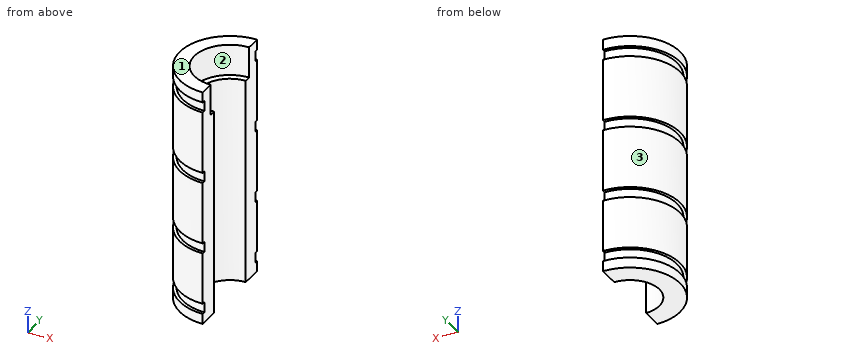
```python
from build123d import *

# Parameters (mm, degrees)
SKETCH1_R           = 24
SKETCH1_R_2         = 14
BOSS_EXTRUDE1_DEPTH = 115
SKETCH2_W           = 30.560484556
SKETCH2_H           = 55.665733052
CUT_EXTRUDE1_DEPTH  = 130
SKETCH3_R           = 17
CUT_EXTRUDE2_DEPTH  = 15
SKETCH4_R           = 29.348690421
SKETCH4_R_2         = 22.5
CUT_EXTRUDE3_DEPTH  = 5
SKETCH5_R           = 32.227537674
SKETCH5_R_2         = 22.5
CUT_EXTRUDE4_DEPTH  = 5
SKETCH6_R           = 32.40953394
SKETCH6_R_2         = 22.5
CUT_EXTRUDE5_DEPTH  = 5
CUT_EXTRUDE6_START  = 5
SKETCH7_R           = 39.356381894
SKETCH7_R_2         = 22.5
CUT_EXTRUDE6_DEPTH  = 5


with BuildPart() as part:
    # Sketch1 → Boss-Extrude1 (new body)
    with BuildSketch(Plane.XY):
        Circle(SKETCH1_R)
        Circle(SKETCH1_R_2, mode=Mode.SUBTRACT)
    extrude(amount=BOSS_EXTRUDE1_DEPTH)

    # Sketch2 → Cut-Extrude1 (cut)
    with BuildSketch(Plane.XY.offset(115)):
        with Locations((15.280242278, -0.503267732)):
            Rectangle(SKETCH2_W, SKETCH2_H)
    extrude(amount=-CUT_EXTRUDE1_DEPTH, mode=Mode.SUBTRACT)

    # Sketch3 → Cut-Extrude2 (cut)
    with BuildSketch(Plane.XY.offset(115)):
        Circle(SKETCH3_R)
    extrude(amount=-CUT_EXTRUDE2_DEPTH, mode=Mode.SUBTRACT)

    # Sketch4 → Cut-Extrude3 (cut)
    with BuildSketch(Plane(origin=(0, 0, 35), x_dir=(-1, 0, 0), z_dir=(0, 0, -1))):
        Circle(SKETCH4_R)
        Circle(SKETCH4_R_2, mode=Mode.SUBTRACT)
    extrude(amount=-CUT_EXTRUDE3_DEPTH, mode=Mode.SUBTRACT)

    # Sketch5 → Cut-Extrude4 (cut)
    with BuildSketch(Plane(origin=(0, 0, 70), x_dir=(-1, 0, 0), z_dir=(0, 0, -1))):
        Circle(SKETCH5_R)
        Circle(SKETCH5_R_2, mode=Mode.SUBTRACT)
    extrude(amount=-CUT_EXTRUDE4_DEPTH, mode=Mode.SUBTRACT)

    # Sketch6 → Cut-Extrude5 (cut)
    with BuildSketch(Plane.XY.offset(105)):
        Circle(SKETCH6_R)
        Circle(SKETCH6_R_2, mode=Mode.SUBTRACT)
    extrude(amount=CUT_EXTRUDE5_DEPTH, mode=Mode.SUBTRACT)

    # Sketch7 → Cut-Extrude6 (cut)
    with BuildSketch(Plane(origin=(0, 0, 10), x_dir=(-1, 0, 0), z_dir=(0, 0, -1)).offset(CUT_EXTRUDE6_START)):
        Circle(SKETCH7_R)
        Circle(SKETCH7_R_2, mode=Mode.SUBTRACT)
    extrude(amount=-CUT_EXTRUDE6_DEPTH, mode=Mode.SUBTRACT)


solid = part.part
```
Geometry: final body of the model. Coordinates: model frame, mm. Face numbers are marked on the shaded views. Give positions to 0.01 mm unless a question says otherwise; leave off trailing zeros. Order: outer loops, then holes, each group sorted by start corner. A loop starts at its lowest first (then second) coordinate and runs counter-clockwise, first axis right, second up. Notation, with made-up numbers: (73, -31.5) -> (111, -31.5) arc R11 ccw to (111, -18.5) -> close; hole circle Ø8 at (79, 32.25). An arc over 180 degrees is marked (long way). Write each question's results on one line, items separated by ' | '. Start each with the question number.
1) Line query: line 1 (Z direction, x = -20, y = -12.5); line 2 (Z direction, x = -12.5, y = -6.5); line 3 (Y direction, x = -12.75, z = 11). Output: solid intervals per line, ascending. Write a range as from..to.
2) Section C-C (y = 20.5). Return loops of the section in (x, z), then the cut area to 3 significant figures.
3) Section B-B (z = 46.5). Return loops of the section in (x, y), then the cut area to 3 significant figures.
4) Section A-A (y = 0). Return loops of the section in (x, z).
5) First-contact query: pin 1 (6 mm diameter, centred on y = 1, z = 99.5, fed in from -X); pin 2 (12 mm diameter, centred on x = -9, y = -2, fed in from -Z); pin 3 (2 mm diameter, centred on x = -3.5, z = 61.5, fed in from -Y); pin 4 (5 mm diameter, centred on x = -12.5, y = 4.5, fed in from +Z). Flat tips, straight axial feed; report the tip coordinate or a pass-through.
6) Draft query along Y for the marked faces 1, 2 and 3. Return one class per face: pulls with the +Y half, pulls with the -Y half, needs draft (parallel to the pull), parting line crosses it, or undercut.
Calculated:
1) line 1: 0..5, 10..35, 40..70, 75..105, 110..115 | line 2: 0..100 | line 3: -20.33..-5.78, 5.78..20.33
2) outline: (-12.48, 0) -> (0, 0) -> (0, 115) -> (-12.48, 115) -> (-12.48, 110) -> (-9.27, 110) -> (-9.27, 105) -> (-12.48, 105) -> (-12.48, 75) -> (-9.27, 75) -> (-9.27, 70) -> (-12.48, 70) -> (-12.48, 40) -> (-9.27, 40) -> (-9.27, 35) -> (-12.48, 35) -> (-12.48, 10) -> (-9.27, 10) -> (-9.27, 5) -> (-12.48, 5) -> close | area: 1,370 mm2
3) outline: (0, -24) -> (0, -14) arc R14 cw to (0, 14) -> (0, 24) arc R24 ccw to start | area: 597 mm2
4) outline: (-24, 0) -> (-14, 0) -> (-14, 100) -> (-17, 100) -> (-17, 115) -> (-24, 115) -> (-24, 110) -> (-22.5, 110) -> (-22.5, 105) -> (-24, 105) -> (-24, 75) -> (-22.5, 75) -> (-22.5, 70) -> (-24, 70) -> (-24, 40) -> (-22.5, 40) -> (-22.5, 35) -> (-24, 35) -> (-24, 10) -> (-22.5, 10) -> (-22.5, 5) -> (-24, 5) -> close
5) pin 1: x = -24 | pin 2: z = 0 | pin 3: y = -23.87 | pin 4: z = 100
6) face 1: needs draft | face 2: undercut | face 3: parting line crosses it
